Can you work these out from the drawing? Everything is in mm from the part's minimum corner. Coordinates: 2 decimals unless noted, no trailing zeros. Order: outer loops, then holes, each group sorted by start corner. A loop starts at its lowest first (then second) coordinate and runs counter-clockwise, first axis right, second up. Notation, with made-up numbers: (-25, -23) - (-17, -23) arc R17 cw to (-17, -14) - close; hole circle Ø10 at (4, 46.5). An arc over 180 degrees is marked (long way). Answer as CSV lines item,"result". Start each with the question number.
Item 1: Imagine slicing it at C-C on y = 25. List the corners of the cut face in (x, z) for me, and give its area (3 significant figures).
Item 2: Imagine slicing it at A-A on z = 165.1. List the corners of the cut face in (x, y) for me.
Item 3: I need wall thicknesses on line 1 (X direction, y = 24, z = 104.5); line 2 (X direction, y = 24, z = 238); line 3 (Z direction, x = 136, y = 10). Which ranges of each line are inside material? Lowest first, please.
Item 4: I'm going to push flat-ended pins straight in: pin 1 (5 mm diameter, centred on x = 180, z = 293.5, fed in from +Y); pin 2 (5 mm diameter, centred on x = 72, y = 15.5, fed in from -Z); pin 3 (3 mm diameter, centred on y = 32, z = 151, fed in from +X) (1 decimal). Where does each tip first touch, or does it pass through?
Item 5: Imagine slicing it at B-B on x = 165.1. List the corners of the cut face in (y, z) for me, and give its area (3 significant figures).
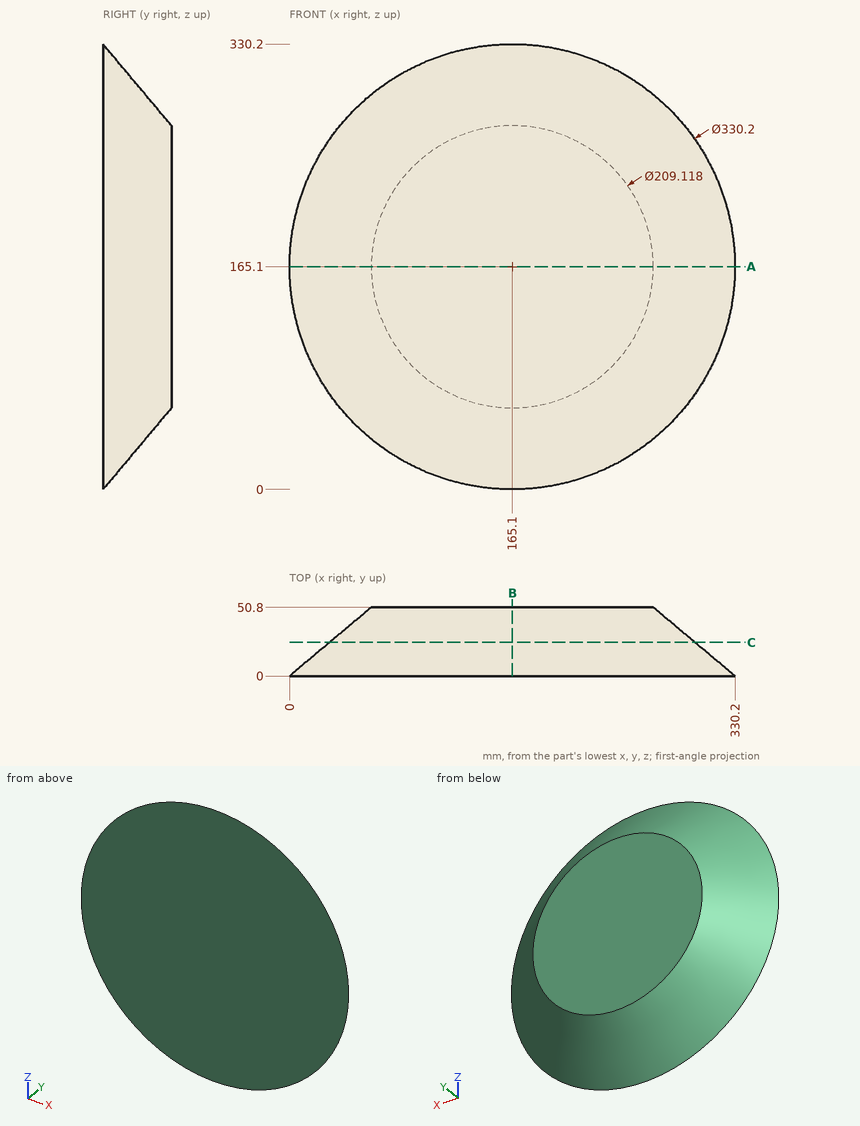
Responses:
1,outline,"circle Ø270.61 at (165.1, 165.1)"
1,area,"57,500 mm^2"
2,outline,"(0, 0) - (330.2, 0) - (269.66, 50.8) - (60.54, 50.8) - close"
3,line 1,"x = 42.79 to 287.41"
3,line 2,"x = 49.7 to 280.5"
3,line 3,"z = 14.71 to 315.49"
4,pin 1,"stops at y = 32.17"
4,pin 2,"stops at z = 47.51"
4,pin 3,"stops at x = 293.1"
5,outline,"(0, 0) - (50.8, 60.54) - (50.8, 269.66) - (0, 330.2) - close"
5,area,"13,700 mm^2"
